The model under review builds one solid part; all positions refer to its coordinate system, in mm. Coordinates: 2 decimals unless noted, no trailing zeros. Write each loop counter-clockwise with the first axis right and the second up, starting at its lowest first coordinate (ties: lowest second). Pieces come first, ordered by that corner, then holes.
```python
from build123d import *

# Parameters (mm, degrees)
SKETCH1_R           = 1.7
SKETCH1_R_2         = 1.27
SKETCH1_R_3         = 1.0922
BOSS_EXTRUDE1_DEPTH = 6.35


with BuildPart() as part:
    # Sketch1 → Boss-Extrude1 (new body)
    with BuildSketch(Plane(origin=(0, 0, 0), x_dir=(1, 0, 0), z_dir=(0, 1, 0))):
        Polygon((32.881906518, 19.245524772), (-0.226160103, 38.099328755), (-33.108066621, 18.853803983), (-32.881906518, -19.245524772), (0.226160103, -38.099328755), (33.108066621, -18.853803983), align=None)
        with Locations(Location((-13.617824536, 23.109102356, 0), (0, 0, 270))):
            Circle(SKETCH1_R, mode=Mode.SUBTRACT)
        with Locations(Location((13.204157431, 23.347933171, 0), (0, 0, 270))):
            Circle(SKETCH1_R, mode=Mode.SUBTRACT)
        with Locations(Location((26.821981967, 0.238830814, 0), (0, 0, 270))):
            Circle(SKETCH1_R, mode=Mode.SUBTRACT)
        with Locations(Location((13.617824536, -23.109102356, 0), (0, 0, 270))):
            Circle(SKETCH1_R, mode=Mode.SUBTRACT)
        with Locations(Location((-13.204157431, -23.347933171, 0), (0, 0, 270))):
            Circle(SKETCH1_R, mode=Mode.SUBTRACT)
        with Locations(Location((-26.821981967, -0.238830814, 0), (0, 0, 270))):
            Circle(SKETCH1_R, mode=Mode.SUBTRACT)
        with Locations(Location((0, 0, 0), (0, 0, 270))):
            Circle(SKETCH1_R_2, mode=Mode.SUBTRACT)
        with Locations(Location((-31.678258679, 18.028303983, 0), (0, 0, 270))):
            Circle(SKETCH1_R_3, mode=Mode.SUBTRACT)
        with Locations(Location((-0.226160103, 36.448328755, 0), (0, 0, 270))):
            Circle(SKETCH1_R_3, mode=Mode.SUBTRACT)
        with Locations(Location((31.452098576, 18.420024772, 0), (0, 0, 270))):
            Circle(SKETCH1_R_3, mode=Mode.SUBTRACT)
        with Locations(Location((31.678258679, -18.028303983, 0), (0, 0, 270))):
            Circle(SKETCH1_R_3, mode=Mode.SUBTRACT)
        with Locations(Location((0.226160103, -36.448328755, 0), (0, 0, 270))):
            Circle(SKETCH1_R_3, mode=Mode.SUBTRACT)
        with Locations(Location((-31.452098576, -18.420024772, 0), (0, 0, 270))):
            Circle(SKETCH1_R_3, mode=Mode.SUBTRACT)
        Polygon((3.715409704, 24.628910363), (7.031797703, 22.753364938), (10.407779468, 28.722863336), (7.091391469, 30.598408761), align=None, mode=Mode.SUBTRACT)
        Polygon((-10.917602296, 28.532975866), (-7.435855918, 22.624540696), (-4.153391934, 24.55884424), (-7.635138312, 30.46727941), align=None, mode=Mode.SUBTRACT)
        Polygon((15.875499033, 17.751910472), (19.191887032, 15.876365047), (22.567868797, 21.845863445), (19.251480798, 23.72140887), align=None, mode=Mode.SUBTRACT)
        Polygon((23.186966894, 9.096815993), (23.22089091, 5.286967024), (30.078619053, 5.348030252), (30.044695037, 9.15787922), align=None, mode=Mode.SUBTRACT)
        Polygon((-19.47155719, 15.532094371), (-16.189093207, 17.466397914), (-19.670839585, 23.374833084), (-22.953303568, 21.440529541), align=None, mode=Mode.SUBTRACT)
        Polygon((23.311354951, -4.872630224), (23.345278966, -8.682479193), (30.203007109, -8.621415965), (30.169083094, -4.811566997), align=None, mode=Mode.SUBTRACT)
        Polygon((19.47155719, -15.532094371), (16.189093207, -17.466397914), (19.670839585, -23.374833084), (22.953303568, -21.440529541), align=None, mode=Mode.SUBTRACT)
        Polygon((7.435855918, -22.624540696), (4.153391934, -24.55884424), (7.635138312, -30.46727941), (10.917602296, -28.532975866), align=None, mode=Mode.SUBTRACT)
        Polygon((-3.715409704, -24.628910363), (-7.031797703, -22.753364938), (-10.407779468, -28.722863336), (-7.091391469, -30.598408761), align=None, mode=Mode.SUBTRACT)
        Polygon((-15.875499033, -17.751910472), (-19.191887032, -15.876365047), (-22.567868797, -21.845863445), (-19.251480798, -23.72140887), align=None, mode=Mode.SUBTRACT)
        Polygon((-23.186966894, -9.096815993), (-23.22089091, -5.286967024), (-30.078619053, -5.348030252), (-30.044695037, -9.15787922), align=None, mode=Mode.SUBTRACT)
        Polygon((-23.311354951, 4.872630224), (-23.345278966, 8.682479193), (-30.203007109, 8.621415965), (-30.169083094, 4.811566997), align=None, mode=Mode.SUBTRACT)
        Polygon((-13.422443502, 20.276025186), (-11.234134179, 21.565560882), (-8.01029494, 16.094787576), (-10.198604263, 14.805251881), align=None, mode=Mode.SUBTRACT)
        Polygon((10.848331148, 21.762189646), (13.059256481, 20.51182603), (9.933347439, 14.984512698), (7.722422107, 16.234876315), align=None, mode=Mode.SUBTRACT)
        Polygon((24.27077465, 1.48616446), (24.29339066, -1.053734852), (17.94364238, -1.110274878), (17.921026369, 1.429624434), align=None, mode=Mode.SUBTRACT)
        Polygon((13.422443502, -20.276025186), (11.234134179, -21.565560882), (8.01029494, -16.094787576), (10.198604263, -14.805251881), align=None, mode=Mode.SUBTRACT)
        Polygon((-10.848331148, -21.762189646), (-13.059256481, -20.51182603), (-9.933347439, -14.984512698), (-7.722422107, -16.234876315), align=None, mode=Mode.SUBTRACT)
        Polygon((-24.27077465, -1.48616446), (-24.29339066, 1.053734852), (-17.94364238, 1.110274878), (-17.921026369, -1.429624434), align=None, mode=Mode.SUBTRACT)
    extrude(amount=-BOSS_EXTRUDE1_DEPTH)


solid = part.part
```
Item 1: Take a section at C-C, the plane z = 32. Write out the cut boundary in (x, y), plus the area to 3 significant figures.
Solved:
outline: (-10.48, -6.35) - (10.65, -6.35) - (10.65, 0) - (-10.48, 0) - close
area: 134 mm2
Item 2: To check wall thickness, follow line 1 along Z through (x, y) = (29, -1.5); line 2 along Z through (x, y) = (25.5, -1); line 3 along Z through (x, y) = (9, -4.75). State the ranges of each line that lie inside material, in increasing order.
Solved:
line 1: z = -21.46 to -9.15, -5.34 to 4.82, 8.63 to 21.26
line 2: z = -23.45 to -9.12, -5.31 to -1.31, 0.83 to 4.85, 8.66 to 23.31
line 3: z = -32.85 to -29.52, -26.23 to -18.49, -15.51 to 15.51, 17.77 to 25.28, 29.66 to 32.96
Item 3: Take a section at B-B, the plane y = -2.25. Count the separate pieces of the cut face and the enclosed holes in it, plus the area to 3 significant figures.
Solved:
separate pieces: 1
enclosed holes: 31
area: 3,280 mm2
Item 4: Mouldability with a two-part tool opening along Z and no side actions: class faces 1 (the face through (9.2, -3.13, 25.62)), 2 (the face through (-16.56, -3.13, 28.54)), 3 (the face through (0, -6.35, 8)) as pulls with the +Z half, pulls with the -Z half, needs draft (parallel to the pull), parting line crosses it, or undercut.
Solved:
face 1: undercut
face 2: pulls with the +Z half
face 3: needs draft
Item 5: For pin 1 (2 mm diameter, centred on x = 31.45, z = -18.42, fed in from +Y); pin 2 (1.5 mm diameter, centred on x = 21.5, y = -3.5, fed in from -Z), all flat-tipped, find the tip position at first contact; note any pin that passes through.
Solved:
pin 1: passes through
pin 2: stops at z = -26.15
Item 6: Take a section at A-A, the plane z = 0. Write out the cut boundary in (x, y).
Solved:
outline: (-33, -6.35) - (-28.51, -6.35) - (-28.51, 0) - (-33, 0) - close; (-25.14, -6.35) - (-24.28, -6.35) - (-24.28, 0) - (-25.14, 0) - close; (-17.93, -6.35) - (-1.27, -6.35) - (-1.27, 0) - (-17.93, 0) - close; (1.27, -6.35) - (17.93, -6.35) - (17.93, 0) - (1.27, 0) - close; (24.28, -6.35) - (25.14, -6.35) - (25.14, 0) - (24.28, 0) - close; (28.51, -6.35) - (33, -6.35) - (33, 0) - (28.51, 0) - close
